Can you work these out from the model? Positions are in its coordinate system, mm. Face numbers are marked on the shaded views. Coordinates: 2 decimals unless noted, no trailing zeros. Order: outer loops, then holes, each group sorted by start corner. A loop starts at its lowest first (then second) coordinate and runs counter-clockwise, first axis right, second up.
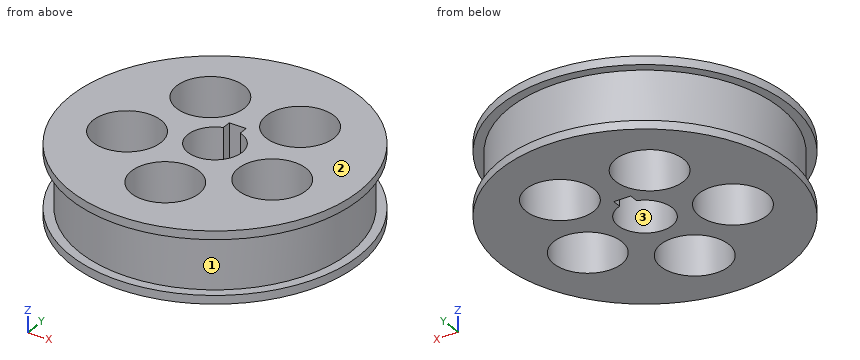
Autodesk Inventor part; units mm, degrees
ref_plane "YZ Plane" through (0, 0, 0) normal (1, 0, 0) x (0, 1, 0)
ref_plane "XZ Plane" through (0, 0, 0) normal (0, 1, 0) x (-1, 0, 0)
ref_plane "XY Plane" through (0, 0, 0) normal (0, 0, 1) x (1, 0, 0)
sketch "Sketch1" plane through (0, 0, 0) normal (0, 0, 1) x (1, 0, 0)
  circle A0 centre (0, 0) radius 42.5
  dimension "d0" = 85
extrude "Extrusion1" add sketch "Sketch1" along normal blind 2.5
sketch "Sketch2" plane through (0, 0, 2.5) normal (0, 0, 1) x (1, 0, 0)
  circle A0 centre (0, 0) radius 39.79
  dimension "d3" = 79.58
extrude "Extrusion2" add sketch "Sketch2" along normal blind 16
sketch "Sketch3" plane through (0, 0, 18.5) normal (0, 0, 1) x (1, 0, 0)
  circle A0 centre (0, 0) radius 42.5
  dimension "d6" = 85
extrude "Extrusion3" add sketch "Sketch3" along normal blind 2.5
sketch "Sketch4" plane through (0, 0, 21) normal (0, 0, 1) x (1, 0, 0)
  circle A0 centre (0, 0) radius 8
  line L0 (-2.5, 5.7) -> (2.5, 5.7)
  line L1 (2.5, 5.7) -> (2.5, 10.3)
  line L2 (2.5, 10.3) -> (-2.5, 10.3)
  line L3 (-2.5, 10.3) -> (-2.5, 5.7)
  line L4 (-2.5, 5.7) -> (2.5, 10.3) construction
  line L5 (2.5, 5.7) -> (-2.5, 10.3) construction
  circle A1 centre (0, 0) radius 22.5
  circle A2 centre (0, -22.5) radius 10
  line L6 (0, 0) -> (0, -22.5)
  line L7 (0, 0) -> (22.5, 0) construction
  circle A3 centre (21.3988, -6.9529) radius 10
  circle A4 centre (13.2252, 18.2029) radius 10
  circle A5 centre (-13.2252, 18.2029) radius 10
  circle A6 centre (-21.3988, -6.9529) radius 10
  point P0 (0, 8)
  dimension "d9" = 16
  dimension "d14" = 45
  dimension "d10" = 5
  dimension "d11" = 4.6
  dimension "d15" = 20
  dimension "d16" = 90
  dimension "d19" = 360
extrude "Extrusion4" cut sketch "Sketch4" against normal blind 21 contours A0 L3 L0 L1 | A2 A1 L6 | L6 A1 A2 | L1 L0 L3 A0 | A0 L3 L2 L1 | A2 A1 | A3 A1 | A1 A3 | A6 A1 | A1 A6 | A4 A1 | A1 A4 | A5 A1 | A1 A5
properties part number "HTD5M 50 Pulley" material "Aluminum 6061"
1. I'm going to push flat-ended pins straight in: pin 1 (5 mm diameter, centred on x = -11, z = 8, fed in from -Y); pin 2 (10 mm diameter, centred on y = -30.5, z = 15, fed in from -X); pin 3 (2.5 mm diameter, centred on x = 0.5, z = 7, fed in from -Y). Where does each tip first touch, or does it pass through?
Completed:
pin 1: stops at y = -38.87
pin 2: stops at x = -32.88
pin 3: stops at y = -39.79
2. Please list where these lines run through material, in increasing order: probe 1 along Y at (x, z) = (0, 4.75); probe 2 along Z at (x, y) = (-35, -23); probe 3 along X at (y, z) = (20.5, 13).
Completed:
probe 1: y = -39.79 to -32.5, -12.5 to -8, 10.3 to 39.79
probe 2: z = 0 to 2.5, 18.5 to 21
probe 3: x = -34.1 to -22.96, -3.49 to 3.49, 22.96 to 34.1
3. Imagine slicing it at A-A on x = 0. Please give me the cut outline in (y, z).
Completed:
outline: (-42.5, 0) - (-32.5, 0) - (-32.5, 21) - (-42.5, 21) - (-42.5, 18.5) - (-39.79, 18.5) - (-39.79, 2.5) - (-42.5, 2.5) - close; (-12.5, 0) - (-8, 0) - (-8, 21) - (-12.5, 21) - close; (10.3, 0) - (42.5, 0) - (42.5, 2.5) - (39.79, 2.5) - (39.79, 18.5) - (42.5, 18.5) - (42.5, 21) - (10.3, 21) - close
4. Thinking about a two-plate mould opening in Y: for the marked faces 1, 2 and 3, which applies, pulls with the +Y half, pulls with the -Y half, needs draft (parallel to the pull), parting line crosses it, or undercut?
Completed:
face 1: parting line crosses it
face 2: needs draft
face 3: undercut
5. Imagine slicing it at D-D on z = 15.25. Please give me the cut outline in (x, y).
Completed:
outline: circle Ø79.58 at (0, 0); hole circle Ø20 at (-21.4, -6.95); hole circle Ø20 at (-13.23, 18.2); hole circle Ø20 at (0, -22.5); hole (-2.5, 7.6) arc R8 ccw (long way) to (2.5, 7.6) - (2.5, 10.3) - (-2.5, 10.3) - close; hole circle Ø20 at (13.23, 18.2); hole circle Ø20 at (21.4, -6.95)
6. Imagine slicing it at B-B on y = -27.5. Please give me the cut outline in (x, z).
Completed:
outline: (-32.4, 0) - (-8.66, 0) - (-8.66, 21) - (-32.4, 21) - (-32.4, 18.5) - (-28.76, 18.5) - (-28.76, 2.5) - (-32.4, 2.5) - close; (8.66, 0) - (32.4, 0) - (32.4, 2.5) - (28.76, 2.5) - (28.76, 18.5) - (32.4, 18.5) - (32.4, 21) - (8.66, 21) - close
7. Imagine slicing it at C-C on y = 0. Please give me the cut outline in (x, z), then the cut area to 3 significant figures.
Completed:
outline: (-42.5, 0) - (-28.59, 0) - (-28.59, 21) - (-42.5, 21) - (-42.5, 18.5) - (-39.79, 18.5) - (-39.79, 2.5) - (-42.5, 2.5) - close; (-14.21, 0) - (-8, 0) - (-8, 21) - (-14.21, 21) - close; (8, 0) - (14.21, 0) - (14.21, 21) - (8, 21) - close; (28.59, 0) - (42.5, 0) - (42.5, 2.5) - (39.79, 2.5) - (39.79, 18.5) - (42.5, 18.5) - (42.5, 21) - (28.59, 21) - close
area: 759 mm2
